Autodesk Inventor part; units mm, degrees
ref_plane "YZ Plane" through (0, 0, 0) normal (1, 0, 0) x (0, 1, 0)
ref_plane "XZ Plane" through (0, 0, 0) normal (0, 1, 0) x (-1, 0, 0)
ref_plane "XY Plane" through (0, 0, 0) normal (0, 0, 1) x (1, 0, 0)
sketch "Sketch1" plane through (0, 0, 0) normal (0, 1, 0) x (-1, 0, 0)
  line L0 (0, 0) -> (200, 0)
  line L1 (200, 0) -> (200, 150)
  line L2 (200, 150) -> (0, 150)
  line L3 (0, 150) -> (0, 0)
  line L4 (110.1274, 0) -> (89.8726, 0)
  line L5 (85.2304, 13.9946) -> (100, 13.9946)
  line L6 (89.8726, 0) -> (84.1428, 12.2875)
  arc A0 (85.2304, 13.9946) -> (84.1428, 12.2875) centre (85.2304, 12.7946) ccw
  line L7 (100, 13.9946) -> (114.7696, 13.9946)
  line L8 (110, 0.2) -> (110, 13.6303) construction
  arc A1 (115.8572, 12.2875) -> (114.7696, 13.9946) centre (114.7696, 12.7946) ccw
  line L9 (115.8572, 12.2875) -> (110.1274, 0)
  arc A2 (114.7696, 136.0054) -> (115.8572, 137.7125) centre (114.7696, 137.2054) ccw
  line L10 (100, 136.0054) -> (114.7696, 136.0054)
  line L11 (115.8572, 137.7125) -> (110.1274, 150)
  line L12 (110, 149.8) -> (110, 136.3697) construction
  line L13 (85.2304, 136.0054) -> (100, 136.0054)
  arc A3 (84.1428, 137.7125) -> (85.2304, 136.0054) centre (85.2304, 137.2054) ccw
  line L14 (110.1274, 150) -> (89.8726, 150)
  line L15 (89.8726, 150) -> (84.1428, 137.7125)
  line L16 (0.2, 85) -> (-13.2303, 85) construction
  line L17 (-13.1946, 75) -> (-13.1946, 89.7696)
  arc A4 (-12.0565, 90.4946) -> (-13.1946, 89.7696) centre (-12.3946, 89.7696) ccw
  line L18 (-12.0565, 90.4946) -> (0, 84.8726)
  line L19 (0, 84.8726) -> (0, 65.1274)
  line L20 (0, 65.1274) -> (-12.0565, 59.5054)
  arc A5 (-13.1946, 60.2304) -> (-12.0565, 59.5054) centre (-12.3946, 60.2304) ccw
  line L21 (-13.1946, 60.2304) -> (-13.1946, 75)
  point P0 (100, 0)
  point P1 (100, 150)
  point P2 (0, 75)
  point P3 (100, 0)
  point P4 (100, 0)
  point P5 (116.3393, 13.7946)
  point P6 (100, 0)
  point P7 (100, 150)
  point P8 (116.3393, 136.2054)
  point P9 (100, 150)
  point P10 (100, 150)
  point P11 (100, 150)
  point P12 (0, 75)
  point P13 (0, 75)
  point P14 (0, 75)
  point P15 (0, 75)
  dimension "d0" = 200
  dimension "d1" = 150
  dimension "d2" = 15
extrude "Extrusion1" add sketch "Sketch1" along normal blind 35 contours L3 L2 L15 A3 L13 L10 A2 L11 L1 L0 L9 A1 L7 L5 A0 L6 | L6 A0 L5 L7 A1 L9 L0 | L2 L11 A2 L10 L13 A3 L15
extrude "Extrusion2" cut sketch "Sketch1" along normal blind 5.2 contours L6 A0 L5 L7 A1 L9 L0 | L2 L11 A2 L10 L13 A3 L15
extrude "Extrusion3" add sketch "Sketch1" along normal blind 4.8 contours L20 A5 L21 L17 A4 L18 L3
sketch "Sketch2" plane through (0, 35, 0) normal (0, 1, 0) x (1, 0, 0)
  line L0 (0, -84.8726) -> (0, -65.1274)
  line L1 (-200, 0) -> (-200, -150)
  circle A0 centre (-100, -75) radius 2.6
  point P0 (0, 0)
  dimension "d9" = 5.2
extrude "Extrusion4" cut sketch "Sketch2" against normal blind 5.2
sketch "Sketch3" plane through (0, 0, 0) normal (0, -1, 0) x (1, 0, 0)
  line L0 (-200, 0) -> (-200, 150)
  line L1 (0, 0) -> (-200, 0)
  line L2 (-200, 150) -> (-130, 150)
  line L3 (-130, 150) -> (-130, 0)
  line L4 (-130, 0) -> (-200, 0)
  line L5 (-200, 0) -> (-200, 150)
  line L6 (0, 150) -> (0, 84.8726)
  line L7 (0, 150) -> (-70, 150)
  line L8 (-70, 150) -> (-70, 100)
  line L9 (-70, 100) -> (0, 100)
  line L10 (0, 100) -> (0, 150)
  line L11 (0, 0) -> (-70, 0)
  line L12 (-70, 0) -> (-70, 50)
  line L13 (-70, 50) -> (0, 50)
  line L14 (0, 50) -> (0, 0)
  dimension "d12" = 70
  dimension "d13" = 70
  dimension "d14" = 50
  dimension "d15" = 70
  dimension "d16" = 50
extrude "Extrusion5" cut sketch "Sketch3" against normal blind 40
fillet "Fillet1" radius 10 8 edges at (0, 17.5, 100) (-70, 17.5, 100) (-70, 17.5, 150) (-130, 17.5, 150) (-130, 17.5, 0) (-70, 17.5, 0) (0, 17.5, 50) (-70, 17.5, 50)
properties part number "Area mh"
Build history of the part. All positions in model axes, mm. A direction names the side the tool comes from. Give positions to 0.01 mm unless a question says otherwise; leave off trailing zeros. Write each loop counter-clockwise with the first axis right and the second up, starting at its lowest first coordinate (ties: lowest second). Pieces come first, ordered by that corner, then holes. Notation, with made-up numbers: (17.5, -2) - (30.5, -2) arc R14 ccw to (30.5, 4) - close; hole circle Ø8 at (35.5, -2.5). An arc over 180 degrees is marked (long way). Use one line per item in the form item = value. Start each with the question number.
1. Band-saw the part on A-A on y = 17.5. Write the cut outline in (x, z).
2. Band-saw the part on D-D on z = 54. Write the cut outline in (x, y).
3. Two-plate mould, pull along X, no slides. Class faces 1 (the face through (-87.048, 2.564, 143.942)), 2 (the face through (-79, 35, 76)), 3 (the face through (-100, 29.8, 75)), 4 (the face through (-130, 17, 76)): released by +X, released by -X, zero draft, split by the parting line, or undercut.
4. Probe line 1 (Z direction, x = -100, y = 33.6); line 2 (X direction, y = 33, z = 75); line 3 (Y direction, x = -100, z = 9). List the from-to ranges inside material, lowest first. Write a range as [from, to].
5. Band-saw the part on B-B on z = 75. Write the cut outline in (x, y), plus the area to 3 significant figures.
6. Band-saw the part on C-C on x = -100. Write the cut outline in (y, z).
7. Drop flat-ended pins along their axis: pin 1 Ø1 at (y, z) = (19, 52.5) entering from +X; pin 2 Ø7 at (x, z) = (-107, 142.5) entering from -Y; pin 3 Ø4 at (x, y) = (-102, 1.5) entering from -Z. Give the stop position or say it passes through.
8. 3-axis set-ups, long thin cutter, end or side, ignore diameter. For faces 5 (the face through (-35, 17, 100)), 6 (the face through (-100.338, 32.436, 72.422)), 7 (the face through (-100, 5.2, 143)): which of +Z, -Z, +X, -X, +Y, -Y reach the whole face in a straight line?
Conclusion:
q1.outline = (-130, 10) arc R10 ccw to (-120, 0) - (-80, 0) arc R10 ccw to (-70, 10) - (-70, 40) arc R10 cw to (-60, 50) - (-10, 50) arc R10 ccw to (0, 60) - (0, 90) arc R10 ccw to (-10, 100) - (-60, 100) arc R10 cw to (-70, 110) - (-70, 140) arc R10 ccw to (-80, 150) - (-120, 150) arc R10 ccw to (-130, 140) - close
q2.outline = (-130, 0) - (-2, 0) - (-2, 35) - (-130, 35) - close
q3.face_1 = undercut
q3.face_2 = zero draft
q3.face_3 = undercut
q3.face_4 = released by -X
q4.line_1 = [0, 72.4], [77.6, 150]
q4.line_2 = [-130, -102.6], [-97.4, 0]
q4.line_3 = [5.2, 35]
q5.outline = (-130, 0) - (13.19, 0) - (13.19, 4.8) - (0, 4.8) - (0, 35) - (-97.4, 35) - (-97.4, 29.8) - (-102.6, 29.8) - (-102.6, 35) - (-130, 35) - close
q5.area = 4,590 mm²
q6.outline = (0, 13.99) - (5.2, 13.99) - (5.2, 0) - (35, 0) - (35, 72.4) - (29.8, 72.4) - (29.8, 77.6) - (35, 77.6) - (35, 150) - (5.2, 150) - (5.2, 136.01) - (0, 136.01) - close
q7.pin_1 = -2.86
q7.pin_2 = 5.2
q7.pin_3 = 13.99
q8.face_5 = +Z, +X, +Y, -Y
q8.face_6 = +Y
q8.face_7 = -Y
